Source: CAD feature listing. Evaluate the final solid. Frame: model axes, mm. Face numbers are marked on the shaded views. A direction names the side the tool comes from. Give positions to 0.01 mm unless a question says otherwise; leave off trailing zeros. Loops run counter-clockwise (first coordinate to the right, second up) from the corner with the lowest first, then second, coordinate; pieces in that order, holes last. Notation, with made-up numbers: M 30,-23 L 86,-23 A7 cw 86,-19 Z; hole C 45,2.5 d4. An arc over 180 degrees is marked long. Put each result on its own line as item: value.
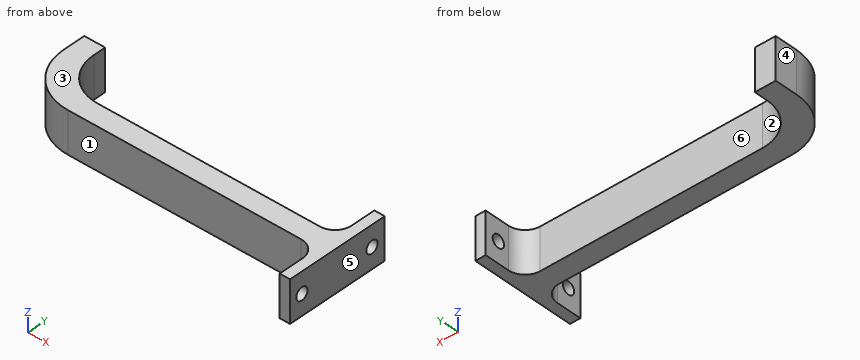
from build123d import *

# Parameters (mm, degrees)
F1_DEPTH = 20
F2_R     = 25
F3_R     = 8
F4_R     = 3
F5_DEPTH = 25
F6_R     = 20


with BuildPart() as f1:
    # F0 (on Top) → F1 (new body)
    with BuildSketch(Plane.XY):
        Polygon((95.607106, 36.108327), (95.607106, 16.108327), (-39.392894, 16.108327), (-39.392894, 42.108327), (-49.392894, 42.108327), (-49.392894, 6.108327), (95.607106, 6.108327), (95.607106, -13.891673), (100.607106, -13.891673), (100.607106, 16.108327), (100.607106, 36.108327), align=None)
    extrude(amount=F1_DEPTH)

    # F2
    f2_edges = [f1.edges().sort_by_distance(p)[0] for p in [
        (-49.392894, 6.108327, 10),
    ]]
    fillet(f2_edges, radius=F2_R)

    # F3
    f3_edges = [f1.edges().sort_by_distance(p)[0] for p in [
        (95.607106, 6.108327, 10),
        (95.607106, 16.108327, 10),
    ]]
    fillet(f3_edges, radius=F3_R)

    # F4 (on face) → F5 (cut)
    with BuildSketch(Plane(origin=(95.607106, 0, 0), x_dir=(0, -1, 0), z_dir=(-1, 0, 0))):
        with Locations((7.59841, 10)):
            Circle(F4_R)
        with Locations((-29.40159, 10)):
            Circle(F4_R)
    extrude(amount=-F5_DEPTH, mode=Mode.SUBTRACT)

    # F6
    f6_edges = [f1.edges().sort_by_distance(p)[0] for p in [
        (-39.392894, 16.108327, 10),
    ]]
    fillet(f6_edges, radius=F6_R)


solid = f1.part
1. Section query A-A (z = 10). Output: boundary loops of the cut face in (x, y), plus the area to 3 significant figures.
Found:
outline: M -49.39,31.11 A25 ccw -24.39,6.11 L 87.61,6.11 A8 cw 95.61,-1.89 L 95.61,-4.6 L 100.61,-4.6 L 100.61,26.4 L 95.61,26.4 L 95.61,24.11 A8 cw 87.61,16.11 L -19.39,16.11 A20 cw -39.39,36.11 L -39.39,42.11 L -49.39,42.11 Z; M 95.61,-13.89 L 100.61,-13.89 L 100.61,-10.6 L 95.61,-10.6 Z; M 95.61,32.4 L 100.61,32.4 L 100.61,36.11 L 95.61,36.11 Z
area: 1,880 mm^2
2. Section query B-B (y = 22). Output: boundary loops of the cut face in (x, z), plus the area to 3 significant figures.
Found:
outline: M -47.67,0 L -33.57,0 L -33.57,20 L -47.67,20 Z; M 95.32,0 L 100.61,0 L 100.61,20 L 95.32,20 Z
area: 388 mm^2
3. Draft query along X for the marked faces 4, 5 and 6. Return one class per face: pulls with the +X half, pulls with the -X half, needs draft (parallel to the pull), parting line crosses it, or undercut.
Found:
face 4: pulls with the -X half
face 5: pulls with the +X half
face 6: undercut
4. Section query C-C (x = 57). Output: boundary loops of the cut face in (y, z).
Found:
outline: M 6.11,0 L 16.11,0 L 16.11,20 L 6.11,20 Z
5. Section query D-D (x = -35). Output: boundary loops of the cut face in (y, z), plus the area to 3 significant figures.
Found:
outline: M 8.47,0 L 23.6,0 L 23.6,20 L 8.47,20 Z
area: 303 mm^2
6. Contact query for flat-ended pins moving along their axis: P1, Ø1.5, axis at x = 29.5, z = 2, coming from the -Y side; P2, Ø2, axis at x = -32, z = 5.5, coming from the +Y side; P3, Ø1, axis at x = 84.5, z = 2, coming from the +Y side. Output: stop coordinate, or through.
Found:
P1: y = 6.11
P2: y = 21.45
P3: y = 16.11
7. Material intervals for line 1 (Y direction, x = 25.5, z = 5); line 2 (X direction, y = -12, z = 2.25); line 3 (X direction, y = 36, z = 11.5), sorted ascending. Write a range as from..to.
Found:
line 1: 6.11..16.11
line 2: 95.61..100.61
line 3: -49.39..-39.39, 95.61..100.61
8. Access query for the marked faces 1, 2 and 3. Directions: +Z, -Z, +X, -X, +Y, -Y. A direction counts if a zero-diameter tool reaches every point of the face in a straight line with its end or side. Return the directions, or none.
Found:
face 1: +Z, -Z, -X, -Y
face 2: +Z, -Z, +Y
face 3: +Z, +X, -X, +Y, -Y
